Input: part model. Units: mm. Frame: model coordinates. Face numbers are marked on the shaded views. A direction names the side the tool comes from. Give positions to 0.01 mm unless a question says otherwise; leave off trailing zeros. Write each loop counter-clockwise with the first axis right and the second up, starting at its lowest first coordinate (ties: lowest second). Pieces come first, ordered by that corner, then holes. Notation, with made-up numbers: (87.25, 16) - (112.25, 16) arc R6 cw to (112.25, 21) - close; hole circle Ø7 at (2.5, -1.75). An arc over 180 degrees is marked (long way). Answer as a JSON object with one key per item and string values. Group by question number.
from build123d import *

# Parameters (mm, degrees)
SKETCH2_W               = 50
SKETCH2_H               = 45
BOSS_EXTRUDE1_DEPTH     = 37.5
BOSS_EXTRUDE2_DEPTH     = 50
CHAMFER2_SIZE           = 2
BOSS_EXTRUDE3_DEPTH     = 10.5
BOSS_EXTRUDE4_DEPTH     = 25
CUT_EXTRUDE2_DEPTH      = 65.143563871
CUT_EXTRUDE2_DEPTH_BACK = 65.143563871
SKETCH10_R              = 2.5
BOSS_EXTRUDE6_DEPTH     = 37.5
SKETCH15_R              = 15.25
BOSS_EXTRUDE8_DEPTH     = 15
SKETCH16_R              = 12.5
BOSS_EXTRUDE9_DEPTH     = 50
SKETCH17_R              = 15.25
BOSS_EXTRUDE10_DEPTH    = 5
SKETCH18_R              = 15
BOSS_EXTRUDE11_DEPTH    = 0.5
SKETCH19_R              = 15.25
BOSS_EXTRUDE12_DEPTH    = 5
SKETCH20_R              = 7.5
SKETCH20_R_2            = 2.5
BOSS_EXTRUDE13_DEPTH    = 10
CUT_EXTRUDE3_DEPTH      = 142.549138883
CUT_EXTRUDE3_DEPTH_BACK = 10
SKETCH21_R              = 7.5


with BuildPart() as part:
    # Sketch2 → Boss-Extrude1 (new body)
    with BuildSketch(Plane.XY):
        Rectangle(SKETCH2_W, SKETCH2_H)
    extrude(amount=-BOSS_EXTRUDE1_DEPTH)

    # Sketch3 → Boss-Extrude2 (add, through all)
    with BuildSketch(Plane(origin=(25, 0, 0), x_dir=(0, 0, -1), z_dir=(1, 0, 0))):
        with BuildLine():
            Line((0, 22.5), (0, -22.5))
            ThreePointArc((0, -22.5), (-4.190481052, 0), (0, 22.5))
        make_face()
        with BuildLine():
            Line((37.5, 22.5), (37.5, -22.5))
            ThreePointArc((37.5, -22.5), (41.690481052, 0), (37.5, 22.5))
        make_face()
    extrude(amount=-BOSS_EXTRUDE2_DEPTH)

    # Chamfer2
    chamfer2_edges = [part.edges().sort_by_distance(p)[0] for p in [
        (25, -22.5, -18.75),
        (-25, -22.5, -18.75),
        (-25, 22.5, -18.75),
        (25, 22.5, -18.75),
    ]]
    chamfer(chamfer2_edges, length=CHAMFER2_SIZE)

    # Sketch7 → Boss-Extrude3 (add)
    with BuildSketch(Plane.XY):
        with BuildLine():
            Line((-21.25, -22.5), (21.25, -22.5))
            ThreePointArc((21.25, -22.5), (0, -43.75), (-21.25, -22.5))
        make_face()
    extrude(amount=-BOSS_EXTRUDE3_DEPTH)

    # Sketch8 → Boss-Extrude4 (add)
    with BuildSketch(Plane(origin=(0, 0, -10.5), x_dir=(-1, 0, 0), z_dir=(0, 0, -1))):
        with BuildLine():
            Line((-10, -22.5), (10, -22.5))
            Line((10, -22.5), (10, -37.5))
            ThreePointArc((10, -37.5), (0, -40.527756377), (-10, -37.5))
            Line((-10, -37.5), (-10, -22.5))
        make_face()
    extrude(amount=BOSS_EXTRUDE4_DEPTH)

    # Sketch10 → Cut-Extrude2 (cut, two sides: drawn at the far end of the back side and taken through both)
    with BuildSketch(Plane(origin=(0, 0, -35.5), x_dir=(-1, 0, 0), z_dir=(0, 0, -1)).offset(-CUT_EXTRUDE2_DEPTH_BACK)):
        with Locations((0, -22.5)):
            Circle(SKETCH10_R)
    extrude(amount=CUT_EXTRUDE2_DEPTH + CUT_EXTRUDE2_DEPTH_BACK, mode=Mode.SUBTRACT)

    # Sketch13 → Boss-Extrude6 (add)
    with BuildSketch(Plane.XY):
        Polygon((23, 22.5), (23, -22.5), (42.5, -17.25), (42.5, 0), (42.5, 17.25), align=None)
    extrude(amount=-BOSS_EXTRUDE6_DEPTH)

    # Sketch15 → Boss-Extrude8 (add)
    with BuildSketch(Plane(origin=(42.5, 0, 0), x_dir=(0, 0, -1), z_dir=(1, 0, 0))):
        with Locations((18.75, 0)):
            Circle(SKETCH15_R)
    extrude(amount=BOSS_EXTRUDE8_DEPTH)

    # Sketch16 → Boss-Extrude9 (add)
    with BuildSketch(Plane(origin=(57.5, 0, 0), x_dir=(0, 0, -1), z_dir=(1, 0, 0))):
        with Locations((18.75, 0)):
            Circle(SKETCH16_R)
    extrude(amount=BOSS_EXTRUDE9_DEPTH)

    # Sketch17 → Boss-Extrude10 (add)
    with BuildSketch(Plane(origin=(107.5, 0, 0), x_dir=(0, 0, -1), z_dir=(1, 0, 0))):
        with Locations((18.75, 0)):
            Circle(SKETCH17_R)
    extrude(amount=BOSS_EXTRUDE10_DEPTH)

    # Sketch18 → Boss-Extrude11 (add)
    with BuildSketch(Plane(origin=(112.5, 0, 0), x_dir=(0, 0, -1), z_dir=(1, 0, 0))):
        with Locations((18.75, 0)):
            Circle(SKETCH18_R)
    extrude(amount=BOSS_EXTRUDE11_DEPTH)

    # Sketch19 → Boss-Extrude12 (add)
    with BuildSketch(Plane(origin=(113, 0, 0), x_dir=(0, 0, -1), z_dir=(1, 0, 0))):
        with Locations((18.75, 0)):
            Circle(SKETCH19_R)
    extrude(amount=BOSS_EXTRUDE12_DEPTH)

    # Sketch20 → Boss-Extrude13 (add)
    with BuildSketch(Plane(origin=(118, 0, 0), x_dir=(0, 0, -1), z_dir=(1, 0, 0))):
        with Locations((18.75, 0)):
            Circle(SKETCH20_R)
        with Locations((18.75, 0)):
            Circle(SKETCH20_R_2, mode=Mode.SUBTRACT)
    extrude(amount=BOSS_EXTRUDE13_DEPTH)

    # Sketch21 → Cut-Extrude3 (cut, two sides: drawn at the far end of the back side and taken through both)
    with BuildSketch(Plane.XY.offset(-CUT_EXTRUDE3_DEPTH_BACK)):
        with Locations((0, -22.5)):
            Circle(SKETCH21_R)
    extrude(amount=CUT_EXTRUDE3_DEPTH + CUT_EXTRUDE3_DEPTH_BACK, mode=Mode.SUBTRACT)


solid = part.part
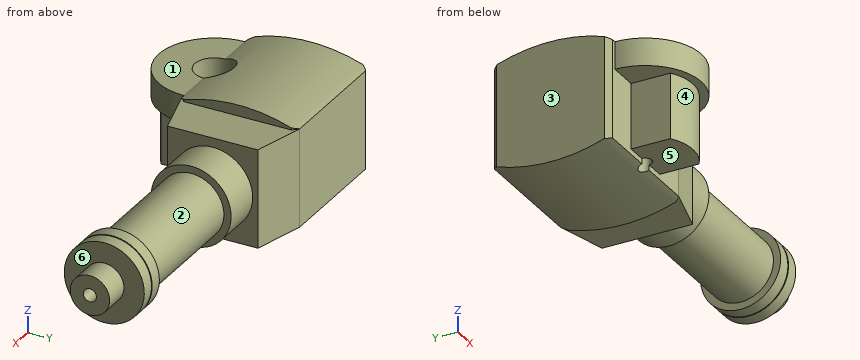
1) Pin query (flat end, axial travel): P1, Ø8, axis at x = 60, y = -6.5, coming from the +Z side; P2, Ø10, axis at x = 10, z = -6.5, coming from the -Y side; P3, Ø6, axis at x = 31.5, y = -8.5, coming from the +Z side. Return the tip coordinate at first contact, or that it passes through.
2) Cut plane A-A on x = 0. Return the cut outline in (y, z), and give its area (3 significant figures).
3) Cut plane C-C on y = -35. Return the cut outline in (x, z).
4) Line query: line 1 along Y through (x, z) = (0, -6.25); line 2 along Y through (x, z) = (0, -19); line 3 along X through (y, z) = (-14, -22.5). Output: solid intervals per line, ascending. Write a range as from..to.
5) Reachability of the marked faces 4, 5 and 6 from +Z, -Z, +X, -X, +Y, -Y: full face, straight path, thin tool, end or side. Return the list, or none.
6) Cut plane B-B on x = 18. Return the cut outline in (y, z), and give its area (3 significant figures).
7) Mould query, pull axis X, two halves, no side actions, for the marked faces 1, 2 and 3. Classes: +X half, -X half, draft (parallel to the pull), parting line (faces both ways), or undercut.
Filled in:
{
 "1": {"P1": "stops at z = -3.88", "P2": "stops at y = -43.15", "P3": "stops at z = 0"},
 "2": {"outline": "(-43.75, -10.5) - (-40.53, -10.5) - (-40.53, -35.5) - (-25, -35.5) - (-25, -10) - (-30, -10) - (-30, 0) - (-43.75, 0) - close; (-20, -38.4) arc R62.5 ccw to (22.5, -37.5) - (22.5, 0) arc R62.5 ccw to (-15, 2.36) - (-15, -10) - (-20, -10) - close", "area": "2,320 mm²"},
 "3": {"outline": "(-17.18, -10.5) - (-10, -10.5) - (-10, -35.5) - (10, -35.5) - (10, -10.5) - (17.18, -10.5) - (17.18, 0) - (-17.18, 0) - close"},
 "4": {"line 1": "y = -43.75..-30, -15..22.5", "line 2": "y = -40.53..-25, -20..22.5", "line 3": "x = -25..57.5, 107.5..118"},
 "5": {"face 4": "-Z, -Y", "face 5": "-Z, +X, -X, -Y", "face 6": "+X"},
 "6": {"outline": "(-33.79, -10.5) - (-22.5, -10.5) - (-22.5, -37.5) arc R62.5 ccw to (22.5, -37.5) - (22.5, 0) arc R62.5 ccw to (-22.5, 0) - (-33.79, 0) - close", "area": "2,060 mm²"},
 "7": {"face 1": "draft", "face 2": "undercut", "face 3": "-X half"}
}
